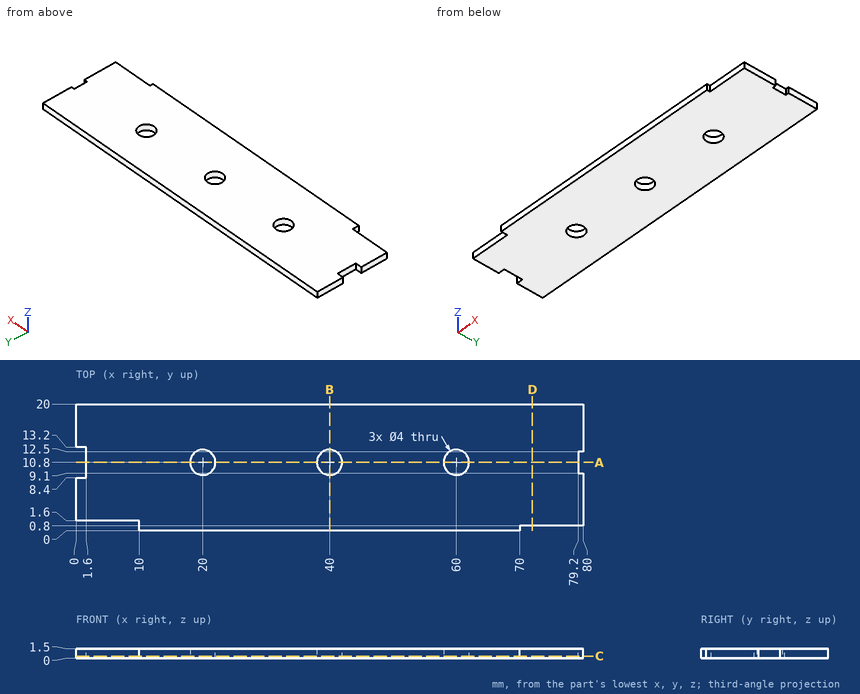
Could you check a few things on this drawing? It's one solid part, dimensions in mm from its lowest x, y, z. Coordinates: 2 decimals unless noted, no trailing zeros. Write each loop counter-clockwise with the first axis right and the second up, starting at its lowest first coordinate (ties: lowest second). Pieces come first, ordered by that corner, then holes. Notation, with made-up numbers: (-30.5, -24) - (17.5, -24) arc R26 cw to (17.5, 1) - close; hole circle Ø11 at (81, -1.5). An arc over 180 degrees is marked (long way). Write item = value, one per line.
1) Suppose I cut it at A-A on y = 10.8. Please give me the cut outline in (x, z).
Result set:
outline = (1.6, 0) - (18, 0) - (18, 1.5) - (1.6, 1.5) - close; (22, 0) - (38, 0) - (38, 1.5) - (22, 1.5) - close; (42, 0) - (58, 0) - (58, 1.5) - (42, 1.5) - close; (62, 0) - (79.2, 0) - (79.2, 1.5) - (62, 1.5) - close
2) Suppose I cut it at C-C on z = 0.35. Please give me the cut outline in (x, y).
Result set:
outline = (0, 1.6) - (10, 1.6) - (10, 0) - (70, 0) - (70, 0.8) - (80, 0.8) - (80, 9.1) - (79.2, 9.1) - (79.2, 12.5) - (80, 12.5) - (80, 20) - (0, 20) - (0, 13.2) - (1.6, 13.2) - (1.6, 8.4) - (0, 8.4) - close; hole circle Ø4 at (20, 10.8); hole circle Ø4 at (40, 10.8); hole circle Ø4 at (60, 10.8)
3) Please list where these lines run through material, in increasing order: line 1 (Y direction, x = 60, z = 0.95); line 2 (X direction, y = 1, z = 1.15); line 3 (Y direction, x = 73.5, z = 0.45). Write a range as [from, to].
Result set:
line_1 = [0, 8.8], [12.8, 20]
line_2 = [10, 80]
line_3 = [0.8, 20]
4) Will this pin go through, and if not, where does the flat tip stop? pin 1 Ø0.8 at (x, z) = (72.5, 1) entering from -Y.
Result set:
pin_1 = 0.8
5) Suppose I cut it at B-B on x = 40. Please give me the cut outline in (y, z), plus the area to 3 significant figures.
Result set:
outline = (0, 0) - (8.8, 0) - (8.8, 1.5) - (0, 1.5) - close; (12.8, 0) - (20, 0) - (20, 1.5) - (12.8, 1.5) - close
area = 24.0 mm2
6) Suppose I cut it at D-D on x = 72. Please give me the cut outline in (y, z), plus the area to 3 significant figures.
Result set:
outline = (0.8, 0) - (20, 0) - (20, 1.5) - (0.8, 1.5) - close
area = 28.8 mm2
